```python
from build123d import *

# Parameters (mm, degrees)
F0_W     = 40
F0_H     = 40
F1_DEPTH = 20
F2_R     = 2
F3_DEPTH = 25
F4_R     = 18
F5_DEPTH = 25
F6_R     = 5


with BuildPart() as f1:
    # F0 (on Top) → F1 (new body)
    with BuildSketch(Plane.XY):
        with Locations((20, 20)):
            Rectangle(F0_W, F0_H)
    extrude(amount=F1_DEPTH)

    # F2 (on face) → F3 (cut)
    with BuildSketch(Plane.XY.offset(20)):
        with Locations((4, 36)):
            Circle(F2_R)
        with Locations((36, 36)):
            Circle(F2_R)
        with Locations((36, 4)):
            Circle(F2_R)
        with Locations((4, 4)):
            Circle(F2_R)
    extrude(amount=-F3_DEPTH, mode=Mode.SUBTRACT)

    # F4 (on face) → F5 (cut)
    with BuildSketch(Plane.XY.offset(20)):
        with Locations((20, 20)):
            Circle(F4_R)
    extrude(amount=-F5_DEPTH, mode=Mode.SUBTRACT)

    # F6
    f6_edges = [f1.edges().sort_by_distance(p)[0] for p in [
        (0, 0, 10),
        (0, 40, 10),
        (40, 40, 10),
        (40, 0, 10),
    ]]
    fillet(f6_edges, radius=F6_R)


solid = f1.part
```
Input: part model. Units: mm. Frame: model coordinates. Coordinates: 2 decimals unless noted, no trailing zeros. Loops run counter-clockwise (first coordinate to the right, second up) from the corner with the lowest first, then second, coordinate; pieces in that order, holes last. Notation, with made-up numbers: M 76.25,67.25 L 122.25,67.25 A25 cw 122.25,87.25 Z; hole C 16,1.5 d5. An arc over 180 degrees is marked long. Answer in a Markdown table with one row per item.
1. Section C-C, the plane y = 36. Output: boundary loops of the cut face in (x, z).
Response:
| item | result |
|---|---|
| outline | M 0.1,0 L 2,0 L 2,20 L 0.1,20 Z; M 6,0 L 11.75,0 L 11.75,20 L 6,20 Z; M 28.25,0 L 34,0 L 34,20 L 28.25,20 Z; M 38,0 L 39.9,0 L 39.9,20 L 38,20 Z |
2. Draft query along X for faces 1 (the cylindrical face through (2.4, 2.8, 10.1)), 2 (the flat face through (20, 40, 10)), 3 (the flat face through (40, 20, 10)). Return one class per face: pulls with the +X half, pulls with the -X half, needs draft (parallel to the pull), parting line crosses it, or undercut.
Response:
| item | result |
|---|---|
| face 1 | undercut |
| face 2 | needs draft |
| face 3 | pulls with the +X half |
3. Material intervals for line 1 (Y direction, x = 4, z = 11); line 2 (Y direction, x = 20, z = 12); line 3 (X direction, y = 24.5, z = 14), sorted ascending.
Response:
| item | result |
|---|---|
| line 1 | y = 0.1 to 2, 6 to 11.75, 28.25 to 34, 38 to 39.9 |
| line 2 | y = 0 to 2, 38 to 40 |
| line 3 | x = 0 to 2.57, 37.43 to 40 |
4. Section A-A, the plane x = 20. Output: boundary loops of the cut face in (y, z), then the cut area to 3 significant figures.
Response:
| item | result |
|---|---|
| outline | M 0,0 L 2,0 L 2,20 L 0,20 Z; M 38,0 L 40,0 L 40,20 L 38,20 Z |
| area | 80.0 mm2 |
5. Section D-D, the plane y = 29. Output: boundary loops of the cut face in (x, z).
Response:
| item | result |
|---|---|
| outline | M 0,0 L 4.41,0 L 4.41,20 L 0,20 Z; M 35.59,0 L 40,0 L 40,20 L 35.59,20 Z |
6. Section B-B, the plane z = 5.25. Output: boundary loops of the cut face in (x, y), then the cut area to 3 significant figures.
Response:
| item | result |
|---|---|
| outline | M 0,5 A5 ccw 5,0 L 35,0 A5 ccw 40,5 L 40,35 A5 ccw 35,40 L 5,40 A5 ccw 0,35 Z; hole C 4,4 d4; hole C 20,20 d36; hole C 4,36 d4; hole C 36,4 d4; hole C 36,36 d4 |
| area | 510 mm2 |
7. First-contact query: pin 1 (3.5 mm diameter, centred on x = 36, y = 4, fed in from +Z). Flat tip, straight axial feed; report the tip coordinate or a pass-through.
Response:
| item | result |
|---|---|
| pin 1 | passes through |
